from build123d import *

# Parameters (mm, degrees)
F0_W     = 8.4
F0_H     = 8.4
F1_DEPTH = 3.3
F2_W     = 8.4
F2_H     = 3.08
F3_DEPTH = 5.1
F5_DEPTH = 25
F6_R     = 2.485
F7_DEPTH = 3.25


with BuildPart() as f1:
    # F0 (on Front) → F1 (new body)
    with BuildSketch(Plane.XZ):
        with Locations((-4.2, 0.163636)):
            Rectangle(F0_W, F0_H)
    extrude(amount=F1_DEPTH)

    # F2 (on face) → F3 (join)
    with BuildSketch(Plane.XZ.offset(3.3)):
        with Locations((-4.2, 0.196881)):
            Rectangle(F2_W, F2_H)
    extrude(amount=F3_DEPTH)

    # F4 (on face) → F5 (cut)
    with BuildSketch(Plane(origin=(0, 0, -1.343119), x_dir=(1, 0, 0), z_dir=(0, 0, -1))):
        with BuildLine():
            Line((-1.293083, 8.4), (-7.072899, 8.4))
            ThreePointArc((-7.072899, 8.4), (-4.182991, 4.484563), (-1.293083, 8.4))
        make_face()
    extrude(amount=-F5_DEPTH, mode=Mode.SUBTRACT)

    # F6 (on face) → F7 (cut)
    with BuildSketch(Plane(origin=(0, 0, 0), x_dir=(-1, 0, 0), z_dir=(0, 1, 0))):
        with Locations((4.167378, 0)):
            Circle(F6_R)
    extrude(amount=-F7_DEPTH, mode=Mode.SUBTRACT)


solid = f1.part
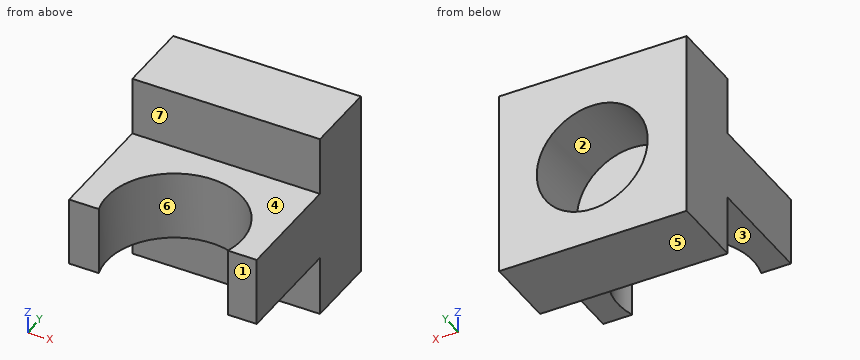
The model under review builds one solid part; all positions refer to its coordinate system, in mm. Face numbers are marked on the shaded views. A direction names the side the tool comes from. Coordinates: 2 decimals unless noted, no trailing zeros. Loops run counter-clockwise (first coordinate to the right, second up) from the corner with the lowest first, then second, coordinate; pieces in that order, holes last. Notation, with made-up numbers: (50, -34.75) -> (58, -34.75) arc R14 ccw to (58, -9.75) -> close; hole circle Ø2 at (-21.5, 20.25). An arc over 180 degrees is marked (long way). Use a Markdown table: item, result. Add a question column.
1. Add section D-D on z = 0.75. Write out the cut boundary in (x, y).
2. Add section C-C on y = -3. Write out the cut boundary in (x, z) (3 decimals).
3. Draft analysis for pull direction Y (two halves, no side actions). For the marked faces 5, 6 and 7, state which applies: pulls with the +Y half, pulls with the -Y half, needs draft (parallel to the pull), parting line crosses it, or undercut.
4. Add section B-B on x = -0.75. Write out the cut boundary in (y, z).
5. Add section A-A on y = -6. Write out the cut boundary in (x, z), plus the area to 3 significant figures.
6. Machinability: for the marked faces 1, 2, 3 and 4, which of the approach directions +Z, -Z, +X, -X, +Y, -Y give a long, thin tool a straight path to every point of the face, cutting with its end or side? Answer none if there is none.
7. Clearance check with flat-ended pins moving along their axes: pin 1 Ø0.8 at (x, z) = (-4.5, -2) entering from -Y; pin 2 Ø2.5 at (x, y) = (-2.5, -5.5) entering from +Z; pin 3 Ø4 at (x, z) = (-4.17, 0) entering from +Y. State where each tip first meets the part, or that it passes through.
8. To check wall thickness, follow line 1 (Y direction, x = -6, z = 3); line 2 (Z direction, x = -3.75, y = -1.5); line 3 (Z direction, x = -1.25, y = -3.5). State the ranges of each line that lie inside material, in increasing order.
Returned:
| question | item | result |
|---|---|---|
| 1 | outline | (-8.4, -8.4) -> (-7.07, -8.4) arc R3.02 cw (long way) to (-1.29, -8.4) -> (0, -8.4) -> (0, 0) -> (-1.8, 0) -> (-1.8, -3.25) -> (-6.54, -3.25) -> (-6.54, 0) -> (-8.4, 0) -> close |
| 2 | outline | (-8.4, -4.036) -> (0, -4.036) -> (0, 4.364) -> (-8.4, 4.364) -> close; hole circle Ø4.97 at (-4.167, 0) |
| 3 | face 5 | needs draft |
| 3 | face 6 | undercut |
| 3 | face 7 | pulls with the -Y half |
| 4 | outline | (-8.4, -1.34) -> (-3.3, -1.34) -> (-3.3, -4.04) -> (0, -4.04) -> (0, 4.36) -> (-3.3, 4.36) -> (-3.3, 1.74) -> (-8.4, 1.74) -> close |
| 5 | outline | (-8.4, -1.34) -> (-6.8, -1.34) -> (-6.8, 1.74) -> (-8.4, 1.74) -> close; (-1.56, -1.34) -> (0, -1.34) -> (0, 1.74) -> (-1.56, 1.74) -> close |
| 5 | area | 9.73 mm² |
| 6 | face 1 | +Z, -Z, +X, -X, -Y |
| 6 | face 2 | +Y |
| 6 | face 3 | -Z, +X, -X, -Y |
| 6 | face 4 | +Z, +X, -X, -Y |
| 7 | pin 1 | stops at y = -3.3 |
| 7 | pin 2 | stops at z = 1.74 |
| 7 | pin 3 | stops at y = -3.25 |
| 8 | line 1 | y = -3.3 to 0 |
| 8 | line 2 | z = -4.04 to -2.45, 2.45 to 4.36 |
| 8 | line 3 | z = -1.34 to 1.74 |
